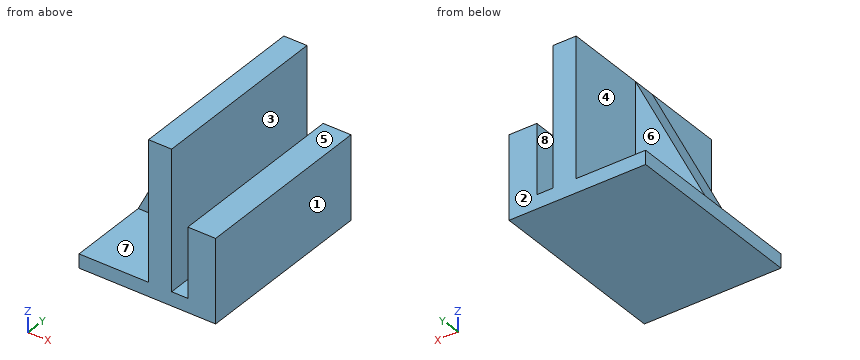
Autodesk Fusion 360 part; units mm, degrees
sketch "Sketch1" plane through (0, 0, 0) normal (0, 0, 1) x (1, 0, 0)
  line L0 (6.75, 20) -> (-6.75, 20)
  line L1 (-6.75, 20) -> (-6.75, -20)
  line L2 (-6.75, -20) -> (6.75, -20)
  line L3 (6.75, -20) -> (6.75, 20)
  line L4 (6.75, 20) -> (-6.75, -20) construction
  line L5 (-6.75, 20) -> (6.75, -20) construction
  line L6 (1.5, -20) -> (-1.5, -20)
  line L7 (-1.5, -20) -> (-1.5, 20)
  line L8 (-1.5, 20) -> (1.5, 20)
  line L9 (1.5, 20) -> (1.5, -20)
  line L10 (1.5, -20) -> (-1.5, 20) construction
  line L11 (-1.5, -20) -> (1.5, 20) construction
  line L12 (1.75, -20) -> (-1.75, -20)
  line L13 (-1.75, -20) -> (-1.75, 20)
  line L14 (-1.75, 20) -> (1.75, 20)
  line L15 (1.75, 20) -> (1.75, -20)
  line L16 (1.75, -20) -> (-1.75, 20) construction
  line L17 (-1.75, -20) -> (1.75, 20) construction
  line L18 (5, -5) -> (-5, -5)
  line L19 (-5, -5) -> (-5, 5)
  line L20 (-5, 5) -> (5, 5)
  line L21 (5, 5) -> (5, -5)
  line L22 (5, -5) -> (-5, 5) construction
  line L23 (-5, -5) -> (5, 5) construction
  line L24 (1.75, -20) -> (6.75, -20)
  line L25 (6.75, -20) -> (6.75, 20)
  line L26 (6.75, 20) -> (1.75, 20)
  line L27 (1.75, 20) -> (1.75, -20)
  line L28 (-6.75, -20) -> (-21.75, -20)
  line L29 (-21.75, -20) -> (-21.75, 20)
  line L30 (-21.75, 20) -> (-6.75, 20)
  line L31 (-6.75, 20) -> (-6.75, -20)
  line L32 (6.75, 20) -> (7.75, 20)
  line L33 (7.75, 20) -> (7.75, -20)
  line L34 (7.75, -20) -> (6.75, -20)
  line L35 (6.75, -20) -> (6.75, 20)
  dimension "d1" = 13.5
  dimension "d2" = 40
  dimension "d3" = 3
  dimension "d4" = 3.5
  dimension "d5" = 40
  dimension "d6" = 10
  dimension "d7" = 10
  dimension "d18" = 5
  dimension "d19" = 15
  dimension "d20" = 40
  dimension "d29" = 1
  dimension "d30" = 40
extrude "Extrude1" add sketch "Sketch1" along normal blind 20 contours L0 L2 L3 L15 L18 L20 L21 L24 L25 L26 L27 L35 | L15 L18 L20 L21 L27 | L0 L1 L2 L13 L18 L19 L20 L31 | L13 L18 L19 L20 makes body 1 at (-1.75, -6.6667, 6.6667) makes body 2 at (6.75, -6.6667, 6.6667)
extrude "Extrude2" add 1 faces at (-3.4167, -6.6667, 20) along direction (0, 0, 1) blind 15 on bodies 1 bodies 1
extrude "Extrude3" add sketch "Sketch1" along normal blind 5 contours L0 L9 L14 L15 L20 L27 | L0 L7 L8 L9 L14 L20 | L9 L15 L18 L20 L27 | L2 L9 L12 L15 L18 L27 | L0 L7 L13 L14 L20 | L7 L9 L18 L20 | L2 L6 L7 L9 L12 L18 | L7 L13 L18 L20 | L2 L7 L12 L13 L18 bodies 1 2
extrude "Extrude4" add sketch "Sketch1" along normal blind 5 contours L0 L2 L3 L15 L18 L20 L21 L24 L25 L26 L27 L35 | L0 L9 L14 L15 L20 L27 | L0 L7 L8 L9 L14 L20 | L2 L9 L12 L15 L18 L27 | L0 L7 L13 L14 L20 | L2 L6 L7 L9 L12 L18 | L0 L1 L2 L13 L18 L19 L20 L31 | L2 L7 L12 L13 L18 bodies 1
extrude "Extrude5" add sketch "Sketch1" along normal blind 5 contours L15 L18 L20 L21 L27 bodies 1
extrude "Extrude6" add sketch "Sketch1" along normal blind 3 contours L1 L28 L29 L30 L31 bodies 1
extrude "Extrude7" cut 1 faces at (0.5833, -6.6667, 5) along direction (0, 0, -1) blind 2 on bodies 1 bodies 1
extrude "Extrude8" cut 1 faces at (5.0833, 6.6667, 20) along direction (0, 0, -1) blind 2 on bodies 1 bodies 1
extrude "Extrude9" cut 1 faces at (-3.4167, -6.6667, 35) along direction (0, 0, -1) blind 2 on bodies 1 bodies 1
extrude "Extrude10" add sketch "Sketch1" along normal blind 18 contours L3 L25 L32 L33 L34 L35 bodies 1
sketch "Sketch2" plane through (0, 0, 0) normal (0, 1, 0) x (1, 0, 0)
  line L0 (-21.75, -3) -> (-6.75, -33)
  line L1 (-6.75, -3) -> (-21.75, -3)
  line L2 (-6.75, -33) -> (-6.75, -3)
  line L3 (-21.75, -3) -> (-6.75, -3)
  point P0 (-21.75, -3)
  point P1 (-6.75, -33)
  point P2 (-6.75, -3)
  point P3 (-6.75, -3)
extrude "Extrude11" add sketch "Sketch2" along normal blind 2.5 bodies 1
extrude "Extrude12" add sketch "Sketch2" against normal blind 2.5 bodies 1
equation "d1 = 3 mm + 0.5 mm + 5 mm + 5 mm"
equation "d8 = 5 mm + 15 mm"
equation "d31 = 3 mm + 15 mm"
CAD build for the part. Positions are in the model's coordinates, mm. Face numbers are marked on the shaded views. A direction names the side the tool comes from. Coordinates: 2 decimals unless noted, no trailing zeros. Write each loop counter-clockwise with the first axis right and the second up, starting at its lowest first coordinate (ties: lowest second). Pieces come first, ordered by that corner, then holes. Notation, with made-up numbers: M 58.25,45 L 68.25,45 A25 ccw 68.25,79 Z; hole C 24.5,42.5 d6. An arc over 180 degrees is marked long. Answer as a JSON object with one key per item and string values. Group by question number.
1) Saw through at A-A (z = 10). Write the cut outline in (x, y), plus the area to 4 significant figures.
2) Saw through at B-B (x = -15.25). Write the cut outline in (y, z).
3) Saw through at D-D (y = -2). Write the cut outline in (x, z), plus the area to 4 significant figures.
4) Tool access for the marked faces 5, 6, 7 and 8: list every direction of +Z, -Z, +X, -X, +Y, -Y with a clear straight run to the whole face (end or side of a thin tool).
5) Wall check: line 1 (X direction, y = -10.5, z = 16.5); line 2 (Z direction, x = -13.25, y = 5.5); line 3 (X direction, y = -17.5, z = 27.5). Give the ranges that are in metal, low to high. Write a range as from..to.
6) Saw through at C-C (z = 26). Write the cut outline in (x, y).
7) Mould opens along X. For the marked faces 1, 2, 3 and 4 say: +X half, -X half, draft (parallel to the pull), parting line (faces both ways), or undercut.
8) Pin check, flat tips, straight feed: pin 1 Ø1.8 at (x, y) = (-0.5, 2) entering from +Z; pin 2 Ø12 at (x, z) = (-10.5, 7.5) entering from -Y; pin 3 Ø1 at (y, z) = (-4, 19.5) entering from -X; pin 4 Ø12 at (x, z) = (-13, 17) entering from +Y. Stop position of each tip, or through.
Values follow:
{
 "1": {"outline": "M -18.25,-2.5 L -6.75,-2.5 L -6.75,-20 L -1.75,-20 L -1.75,20 L -6.75,20 L -6.75,2.5 L -18.25,2.5 Z; M 1.75,-20 L 7.75,-20 L 7.75,20 L 1.75,20 Z", "area": "497.5 mm2"},
 "2": {"outline": "M -20,0 L 20,0 L 20,3 L 2.5,3 L 2.5,16 L -2.5,16 L -2.5,3 L -20,3 Z"},
 "3": {"outline": "M -21.75,0 L 7.75,0 L 7.75,18 L 1.75,18 L 1.75,3 L -1.75,3 L -1.75,33 L -6.75,33 L -21.75,3 Z", "area": "553.5 mm2"},
 "4": {"face 5": "+Z, +X, +Y, -Y", "face 6": "+Z, -X, +Y", "face 7": "+Z, -X, -Y", "face 8": "+Z, +Y, -Y"},
 "5": {"line 1": "x = -6.75..-1.75, 1.75..7.75", "line 2": "z = 0..3", "line 3": "x = -6.75..-1.75"},
 "6": {"outline": "M -10.25,-2.5 L -6.75,-2.5 L -6.75,-20 L -1.75,-20 L -1.75,20 L -6.75,20 L -6.75,2.5 L -10.25,2.5 Z"},
 "7": {"face 1": "+X half", "face 2": "draft", "face 3": "undercut", "face 4": "-X half"},
 "8": {"pin 1": "stops at z = 3", "pin 2": "stops at y = -20", "pin 3": "stops at x = -6.75", "pin 4": "stops at y = 2.5"}
}
